Read the model definition and answer for the solid it produces. Units are mm, in the model's axes. A direction names the side the tool comes from. Coordinates: 2 decimals unless noted, no trailing zeros. Order: outer loops, then holes, each group sorted by start corner. A loop starts at its lowest first (then second) coordinate and runs counter-clockwise, first axis right, second up. Notation, with made-up numbers: (5.5, -23.5) - (25.5, -23.5) arc R31 cw to (25.5, 12.5) - close; hole circle Ø10 at (-2, 34.5). An arc over 180 degrees is marked (long way). Use one line per item in the form item = value.
```python
from build123d import *

# Parameters (mm, degrees)
F0_W     = 177.8
F0_H     = 76.2
F1_DEPTH = 50.8
F3_T     = -2.54


# Not quite as in the source:
# - the program builds the solid bodies; features that only make, move or delete a surface that nothing else refers to are left out


with BuildPart() as f1:
    # F0 (on Front) → F1 (new body)
    with BuildSketch(Plane.XZ):
        Rectangle(F0_W, F0_H)
    extrude(amount=F1_DEPTH)

    # F3
    f3_openings = [f1.faces().sort_by_distance(p)[0] for p in [
        (0, -50.8, 0),
    ]]
    offset(amount=F3_T, openings=f3_openings)


solid = f1.part
```
(1) Given pin 1 Ø2 at (x, z) = (48, -25) entering from -Y, flat-ended and moving along its own axis, determine where the tip first touches the part or whether it passes through.
Answer list:
pin_1 = -2.54
(2) The mould has two halves that part along Z. Classify faces 1 (the flat face through (0, -50.8, 37)), 2 (the flat face through (-1, -26, -35.56)), 3 (the flat face through (-1, -25, -38.1)): +Z half, -Z half, draft (parallel to the pull), parting line (faces both ways), or undercut.
Answer list:
face_1 = draft
face_2 = undercut
face_3 = -Z half
(3) Straight lines are drawn through the part: L1, parallel to X at y = -36.5, z = 9.5; L2, parallel to Z at x = 50, y = -18.5; L3, parallel to Y at x = 10, z = 33.5. For each, find the intervals that lie inside material, in ascending order.
Answer list:
L1 = -88.9 to -86.36, 86.36 to 88.9
L2 = -38.1 to -35.56, 35.56 to 38.1
L3 = -2.54 to 0
(4) Section A-A, the plane y = -32.5 is taken. Write down the section's boundary in (x, z), then the cut area to 3 significant figures.
Answer list:
outline = (-88.9, -38.1) - (88.9, -38.1) - (88.9, 38.1) - (-88.9, 38.1) - close; hole (-86.36, -35.56) - (86.36, -35.56) - (86.36, 35.56) - (-86.36, 35.56) - close
area = 1,260 mm2
(5) Which of the six approach directions +Z, -Z, +X, -X, +Y, -Y give full straight-line access (tool end or side, diameter ignored) to faces 4 (the flat face through (-1, -2.54, 0)), 5 (the flat face through (-1, -25, 38.1))?
Answer list:
face_4 = -Y
face_5 = +Z, +X, -X, +Y, -Y
(6) Section C-C, the plane z = -16.5 is taken. Write down the section's boundary in (x, y), then the cut area to 3 significant figures.
Answer list:
outline = (-88.9, -50.8) - (-86.36, -50.8) - (-86.36, -2.54) - (86.36, -2.54) - (86.36, -50.8) - (88.9, -50.8) - (88.9, 0) - (-88.9, 0) - close
area = 697 mm2
(7) Section B-B, the plane x = 49 is taken. Write down the section's boundary in (y, z), then the cut area to 3 significant figures.
Answer list:
outline = (-50.8, -38.1) - (0, -38.1) - (0, 38.1) - (-50.8, 38.1) - (-50.8, 35.56) - (-2.54, 35.56) - (-2.54, -35.56) - (-50.8, -35.56) - close
area = 439 mm2
